Geometry: final body of the model. Coordinates: model frame, mm. A direction names the side the tool comes from. Give positions to 0.01 mm unless a question says otherwise; leave off trailing zeros. Loops run counter-clockwise (first coordinate to the right, second up) from the corner with the lowest first, then second, coordinate; pieces in that order, holes last. Notation, with made-up numbers: (-27, 9.25) -> (19, 9.25) arc R22 cw to (19, 16.25) -> close; hole circle Ø2 at (40.5, 77). An arc over 180 degrees is marked (long way). Answer in a Markdown table with one row per item. Add a question column.
1) Draft query along Z for faces 3 (the flat face through (-23.292, 17, 0)), 4 (the flat face through (25.4, 17, 0)), 5 (the flat face through (0, 17, -25.4)). Return one class per face: +Z half, -Z half, draft (parallel to the pull), parting line (faces both ways), or undercut.
2) Section query B-B (y = 21). Return the cut outline in (x, z).
3) Section query C-C (z = 5.5). Return the cut outline in (x, y) (3 decimals), plus the area to 3 significant figures.
4) Section query A-A (x = 20.5). Return the cut outline in (y, z) (3 decimals).
5) Access query for faces 1 (the cylindrical face through (22.66, 17.22, -22.69)), 2 (the cylindrical face through (24.2, 17.22, 24.13)). Directions: +Z, -Z, +X, -X, +Y, -Y. A direction counts if a zero-diameter tool reaches every point of the face in a straight line with its end or side. Return the directions, or none.
6) Line query: line 1 (Z direction, x = 3.5, y = 7); line 2 (Z direction, x = 22.5, y = 28). Output: solid intervals per line, ascending. Write a range as from..to.
Solid Edge part; units mm, degrees
sketch "Sketch1" plane through (0, 0, 0) normal (0, -1, 0) x (1, 0, 0)
  arc A0 (-23.2918, -21.1836) -> (-21.1836, -23.2918) centre (-21.1836, -21.1836) ccw
  line L0 (-21.1836, -23.2918) -> (21.1836, -23.2918)
  arc A1 (21.1836, -23.2918) -> (23.2918, -21.1836) centre (21.1836, -21.1836) ccw
  line L1 (23.2918, -21.1836) -> (23.2918, 21.1836)
  arc A2 (23.2918, 21.1836) -> (21.1836, 23.2918) centre (21.1836, 21.1836) ccw
  line L2 (21.1836, 23.2918) -> (-21.1836, 23.2918)
  arc A3 (-21.1836, 23.2918) -> (-23.2918, 21.1836) centre (-21.1836, 21.1836) ccw
  line L3 (-23.2918, 21.1836) -> (-23.2918, -21.1836)
  arc A4 (-25.4, -21.1836) -> (-21.1836, -25.4) centre (-21.1836, -21.1836) ccw
  line L4 (-21.1836, -25.4) -> (21.1836, -25.4)
  arc A5 (21.1836, -25.4) -> (25.4, -21.1836) centre (21.1836, -21.1836) ccw
  line L5 (25.4, -21.1836) -> (25.4, 21.1836)
  arc A6 (25.4, 21.1836) -> (21.1836, 25.4) centre (21.1836, 21.1836) ccw
  line L6 (21.1836, 25.4) -> (-21.1836, 25.4)
  arc A7 (-21.1836, 25.4) -> (-25.4, 21.1836) centre (-21.1836, 21.1836) ccw
  line L7 (-25.4, 21.1836) -> (-25.4, -21.1836)
extrude "Protrusion1" add sketch "Sketch1" against normal blind 34.925
Evaluation:
| question | item | result |
|---|---|---|
| 1 | face 3 | undercut |
| 1 | face 4 | draft |
| 1 | face 5 | -Z half |
| 2 | outline | (-25.4, -21.18) arc R4.22 ccw to (-21.18, -25.4) -> (21.18, -25.4) arc R4.22 ccw to (25.4, -21.18) -> (25.4, 21.18) arc R4.22 ccw to (21.18, 25.4) -> (-21.18, 25.4) arc R4.22 ccw to (-25.4, 21.18) -> close; hole (-23.29, -21.18) arc R2.11 ccw to (-21.18, -23.29) -> (21.18, -23.29) arc R2.11 ccw to (23.29, -21.18) -> (23.29, 21.18) arc R2.11 ccw to (21.18, 23.29) -> (-21.18, 23.29) arc R2.11 ccw to (-23.29, 21.18) -> close |
| 3 | outline | (-25.4, 0) -> (-23.292, 0) -> (-23.292, 34.925) -> (-25.4, 34.925) -> close; (23.292, 0) -> (25.4, 0) -> (25.4, 34.925) -> (23.292, 34.925) -> close |
| 3 | area | 147 mm² |
| 4 | outline | (0, -25.4) -> (34.925, -25.4) -> (34.925, -23.292) -> (0, -23.292) -> close; (0, 23.292) -> (34.925, 23.292) -> (34.925, 25.4) -> (0, 25.4) -> close |
| 5 | face 1 | +Y, -Y |
| 5 | face 2 | +Z, +X, +Y, -Y |
| 6 | line 1 | -25.4..-23.29, 23.29..25.4 |
| 6 | line 2 | -25.19..-22.83, 22.83..25.19 |
